```python
from build123d import *

# Parameters (mm, degrees)
SKETCH1_R           = 18
BOSS_EXTRUDE1_DEPTH = 61
SKETCH2_W           = 39.528935746
SKETCH2_H           = 14.130439677
CUT_EXTRUDE1_DEPTH  = 54
SKETCH3_W           = 60
SKETCH3_H           = 15.7
BOSS_EXTRUDE2_DEPTH = 9
SKETCH4_R           = 3.5
CUT_EXTRUDE2_DEPTH  = 10
LPATTERN1_COUNT     = 2
LPATTERN1_PITCH     = 44
SKETCH6_R           = 5
CUT_EXTRUDE3_DEPTH  = 100


with BuildPart() as part:
    # Sketch1 → Boss-Extrude1 (new body)
    with BuildSketch(Plane.XY):
        Circle(SKETCH1_R)
    extrude(amount=BOSS_EXTRUDE1_DEPTH)

    # Sketch2 → Cut-Extrude1 (cut)
    with BuildSketch(Plane.XY.offset(61)):
        with Locations((2.474682956, 14.065219839)):
            Rectangle(SKETCH2_W, SKETCH2_H)
    extrude(amount=-CUT_EXTRUDE1_DEPTH, mode=Mode.SUBTRACT)

    # Sketch3 → Boss-Extrude2 (add)
    with BuildSketch(Plane.XY.offset(61)):
        with Locations((0, -12.16286005)):
            Rectangle(SKETCH3_W, SKETCH3_H)
    extrude(amount=-BOSS_EXTRUDE2_DEPTH)

    # Sketch4 → Cut-Extrude2 (cut)
    with BuildSketch(Plane(origin=(0, 0, 52), x_dir=(-1, 0, 0), z_dir=(0, 0, -1))):
        with Locations((-22, -11.51286005)):
            Circle(SKETCH4_R)
    cut_extrude2 = extrude(amount=-CUT_EXTRUDE2_DEPTH, mode=Mode.SUBTRACT)

    # LPattern1: Cut-Extrude2 ×2
    with Locations(*[(-i * LPATTERN1_PITCH, 0, 0) for i in range(1, LPATTERN1_COUNT)]):
        add(cut_extrude2, mode=Mode.SUBTRACT)

    # Sketch6 → Cut-Extrude3 (cut)
    with BuildSketch(Plane(origin=(0, 0, 0), x_dir=(-1, 0, 0), z_dir=(0, 0, -1))):
        Circle(SKETCH6_R)
    extrude(amount=-CUT_EXTRUDE3_DEPTH, mode=Mode.SUBTRACT)


solid = part.part
```
Design review of the part built by this model. Coordinates are the model's own, in mm. A direction names the side the tool comes from. Coordinates: 2 decimals unless noted, no trailing zeros. Loops run counter-clockwise (first coordinate to the right, second up) from the corner with the lowest first, then second, coordinate; pieces in that order, holes last. Notation, with made-up numbers: (-7.75, -26.5) -> (51.25, -26.5) arc R25 ccw to (51.25, 7.5) -> close; hole circle Ø6 at (46, 60). An arc over 180 degrees is marked (long way). Answer as a JSON object with one key per item and string values.
Q1. Take a section at C-C on y = -10.5. Give the boundary of the cut face in (x, z), plus the area to 3 significant figures.
Answer block:
{"outline": "(-30, 52) -> (-25.35, 52) -> (-25.35, 61) -> (-30, 61) -> close; (-18.65, 52) -> (-14.62, 52) -> (-14.62, 0) -> (14.62, 0) -> (14.62, 52) -> (18.65, 52) -> (18.65, 61) -> (-18.65, 61) -> close; (25.35, 52) -> (30, 52) -> (30, 61) -> (25.35, 61) -> close", "area": "1,940 mm^2"}
Q2. To check wall thickness, follow L1, parallel to Y at x = 22, z = 55; L2, parallel to Y at x = 0, z = 29; L3, parallel to Y at x = -9, z = 53. State the ranges of each line that lie inside material, in increasing order.
Answer block:
{"L1": "y = -20.01 to -15.01, -8.01 to -4.31", "L2": "y = -18 to -5, 5 to 7", "L3": "y = -20.01 to 7"}
Q3. Tool access review of faces 4 (the cylindrical face through (1.08, -4.88, 30.07)), 5 (the flat face through (0, 11, 7)): name each direction out of +Z, -Z, +X, -X, +Y, -Y from which nothing blocks a thin tool from reaching the whole face with its end or side.
Answer block:
{"face 4": "+Z, -Z", "face 5": "+Z, +X, -X, +Y"}
Q4. Take a section at B-B on x = -22. Give the boundary of the cut face in (y, z).
Answer block:
{"outline": "(-20.01, 52) -> (-15.01, 52) -> (-15.01, 61) -> (-20.01, 61) -> close; (-8.01, 52) -> (-4.31, 52) -> (-4.31, 61) -> (-8.01, 61) -> close"}
Q5. Take a section at D-D on z = 19. Give the boundary of the cut face in (x, y).
Answer block:
{"outline": "(-16.58, 7) arc R18 ccw (long way) to (16.58, 7) -> close; hole circle Ø10 at (0, 0)"}
Q6. The part is to be moulded in two halves that separate along X. For faces 1 (the cylindrical face through (-25.233, -12.853, 56.437)), 2 (the flat face through (0, -19, 52)), 3 (the cylindrical face through (-3.902, -17.572, 23.295)), say which applies: +X half, -X half, draft (parallel to the pull), parting line (faces both ways), or undercut.
Answer block:
{"face 1": "undercut", "face 2": "draft", "face 3": "parting line"}
Q7. Take a section at A-A on y = 0. Give the boundary of the cut face in (x, z).
Answer block:
{"outline": "(-18, 0) -> (-5, 0) -> (-5, 61) -> (-18, 61) -> close; (5, 0) -> (18, 0) -> (18, 61) -> (5, 61) -> close"}
Q8. Clearance check with flat-ended pins moving along their axes: pin 1 Ø8 at (y, z) = (-11, 31) entering from +X; pin 2 Ø16.5 at (x, z) = (8, 36) entering from +Y; pin 3 Ø9 at (x, y) = (-6.5, 12) entering from +Z; pin 4 Ø6 at (x, y) = (0, 0) entering from +Z. State where each tip first meets the part, or that it passes through.
Answer block:
{"pin 1": "stops at x = 16.58", "pin 2": "stops at y = 7", "pin 3": "stops at z = 7", "pin 4": "passes through"}
